CAD build for the part. Positions are in the model's coordinates, mm. A direction names the side the tool comes from. Give positions to 0.01 mm unless a question says otherwise; leave off trailing zeros. Write each loop counter-clockwise with the first axis right and the second up, starting at its lowest first coordinate (ties: lowest second). Pieces come first, ordered by that corner, then holes. Notation, with made-up numbers: (10.5, 37) - (42.5, 37) arc R16 ccw to (42.5, 65) - close; hole circle Ø11 at (4.25, 59). An arc over 180 degrees is marked (long way). Answer as a JSON object with one key per item and string values.
from build123d import *

# Parameters (mm, degrees)
SKETCH2_W           = 30
SKETCH2_H           = 20
BOSS_EXTRUDE1_DEPTH = 2
SKETCH3_R           = 2.5
BOSS_EXTRUDE2_DEPTH = 2


with BuildPart() as part:
    # Sketch2 → Boss-Extrude1 (new body)
    with BuildSketch(Plane.ZY.offset(20)):
        Rectangle(SKETCH2_W, SKETCH2_H)
    extrude(amount=BOSS_EXTRUDE1_DEPTH)

    # Sketch3 → Boss-Extrude2 (add)
    with BuildSketch(Plane(origin=(0, 10, 0), x_dir=(1, 0, 0), z_dir=(0, 1, 0))):
        with BuildLine():
            Line((-22, -15), (-22, 15))
            Line((-22, 15), (-30.660254038, 10))
            Line((-30.660254038, 10), (-38.424825391, -18.977774789))
            Line((-38.424825391, -18.977774789), (-38.424825391, -48.977774789))
            ThreePointArc((-38.424825391, -48.977774789), (-33.424825391, -53.977774789), (-28.424825391, -48.977774789))
            Line((-28.424825391, -48.977774789), (-28.424825391, -20.294299765))
            Line((-28.424825391, -20.294299765), (-27.006222045, -15))
            Line((-27.006222045, -15), (-22, -15))
        make_face()
        with Locations(Location((-33.424825391, -48.977774789, 0), (0, 0, 270))):
            Circle(SKETCH3_R, mode=Mode.SUBTRACT)
        with Locations(Location((-33.424825391, -22.229962666, 0), (0, 0, 270))):
            Circle(SKETCH3_R, mode=Mode.SUBTRACT)
    boss_extrude2 = extrude(amount=-BOSS_EXTRUDE2_DEPTH)

    # Mirror1: Boss-Extrude2 across plane
    add(boss_extrude2.mirror(Plane(origin=(0, 0, 0), x_dir=(0, 0, 1), z_dir=(0, -1, 0))))


solid = part.part
(1) Flat gauge pins, fed straight in: P1, Ø5, axis at y = 0, z = 16, coming from the -X side; P2, Ø1.6, axis at y = 9, z = 36.5, coming from the +X side; P3, Ø4, axis at x = -33.42, z = 22.23, coming from the +Y side; P4, Ø7.5, axis at x = -23.5, y = 2.5, coming from the +Z side. Where does each tip first touch, or does it go through?
Answer key:
{"P1": "stops at x = -22", "P2": "stops at x = -28.42", "P3": "passes through", "P4": "stops at z = 15"}
(2) 3-axis set-ups, long thin cutter, end or side, ignore diameter. For faces 3 (the face through (-38.425, -9, 34)), 4 (the face through (-21, 0, 15)), 5 (the face through (-22, 0, 0)): which of +Z, -Z, +X, -X, +Y, -Y reach the whole face in a straight line?
Answer key:
{"face 3": "+Z, -Z, -X, +Y, -Y", "face 4": "+Z, +X, +Y, -Y", "face 5": "+Z, -Z, -X"}
(3) Probe L1, parallel to Y at x = -32.75, z = 6; L2, parallel to X at y = -0.75, z = -9.5; L3, parallel to X at y = 9.25, z = 39. List the from-to ranges inside material, lowest first. Write a range as [from, to].
Answer key:
{"L1": "y = [-10, -8], [8, 10]", "L2": "x = [-22, -20]", "L3": "x = [-38.42, -28.42]"}
(4) Pull direction Y, two halves, no side cores. Call faces 1 (the face through (-30, 8, 19)), 2 (the face through (-34.49, 9.01, 4.29)): pulls with the +Y half, pulls with the -Y half, needs draft (parallel to the pull), parting line crosses it, or undercut.
Answer key:
{"face 1": "undercut", "face 2": "needs draft"}
(5) Saw through at D-D, the plane z = 7.5. Give the cut face in (x, y).
Answer key:
{"outline": "(-35.35, -10) - (-20, -10) - (-20, 10) - (-35.35, 10) - (-35.35, 8) - (-22, 8) - (-22, -8) - (-35.35, -8) - close"}
(6) Saw through at B-B, the plane x = -23. Give the cut face in (y, z).
Answer key:
{"outline": "(-10, -14.42) - (-8, -14.42) - (-8, 15) - (-10, 15) - close; (8, -14.42) - (10, -14.42) - (10, 15) - (8, 15) - close"}
(7) Saw through at C-C, the plane z = 22.5. Give the cut face in (x, y), and give its area (3 significant figures).
Answer key:
{"outline": "(-38.42, -10) - (-35.91, -10) - (-35.91, -8) - (-38.42, -8) - close; (-38.42, 8) - (-35.91, 8) - (-35.91, 10) - (-38.42, 10) - close; (-30.94, -10) - (-28.42, -10) - (-28.42, -8) - (-30.94, -8) - close; (-30.94, 8) - (-28.42, 8) - (-28.42, 10) - (-30.94, 10) - close", "area": "20.1 mm²"}
(8) Saw through at A-A, the plane z = 41.5. Give the cut face in (x, y), and give its area (3 significant figures).
Answer key:
{"outline": "(-38.42, -10) - (-28.42, -10) - (-28.42, -8) - (-38.42, -8) - close; (-38.42, 8) - (-28.42, 8) - (-28.42, 10) - (-38.42, 10) - close", "area": "40.0 mm²"}
